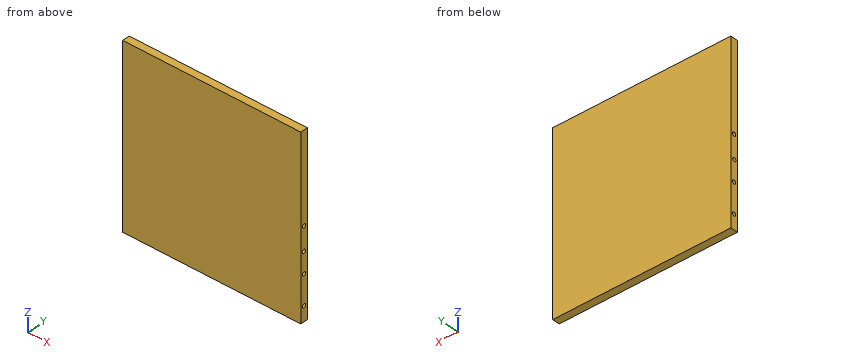
from build123d import *

# Parameters (mm, degrees)
SKETCH2_W               = 304.8
SKETCH2_H               = 304.8
BOSS_EXTRUDE1_DEPTH     = 12.7
SKETCH3_R               = 3.175
CUT_EXTRUDE1_DEPTH      = 343.16151121
SKETCH4_R               = 3.175
CUT_EXTRUDE2_DEPTH      = 343.16151121
CUT_EXTRUDE7_DEPTH      = 343.16151121
CUT_EXTRUDE7_DEPTH_BACK = 343.16151121
SKETCH5_R               = 3.175
CUT_EXTRUDE8_DEPTH      = 343.16151121
CUT_EXTRUDE8_DEPTH_BACK = 343.16151121
SKETCH6_R               = 3.175
SCALE1_SCALE            = 1.5


with BuildPart() as part:
    # Sketch2 → Boss-Extrude1 (new body)
    with BuildSketch(Plane(origin=(0, 0, 0), x_dir=(1, 0, 0), z_dir=(0, 1, 0))):
        with Locations((-98.332011444, 2.55215311)):
            Rectangle(SKETCH2_W, SKETCH2_H)
    extrude(amount=BOSS_EXTRUDE1_DEPTH)

    # Sketch3 → Cut-Extrude1 (cut, through all)
    with BuildSketch(Plane(origin=(54.067988556, 0, 0), x_dir=(0, 0, -1), z_dir=(1, 0, 0))):
        with Locations((2.55215311, 6.35)):
            Circle(SKETCH3_R)
    extrude(amount=-CUT_EXTRUDE1_DEPTH, mode=Mode.SUBTRACT)

    # Sketch4 → Cut-Extrude2 (cut, through all)
    with BuildSketch(Plane.ZY.offset(250.732011444)):
        with Locations((-42.726167629, 5.894382634)):
            Circle(SKETCH4_R)
    extrude(amount=-CUT_EXTRUDE2_DEPTH, mode=Mode.SUBTRACT)

    # Sketch5 → Cut-Extrude7 (cut, two sides: drawn at the far end of the back side and taken through both)
    with BuildSketch(Plane.ZY.offset(250.732011444).offset(-CUT_EXTRUDE7_DEPTH_BACK)):
        with Locations((-78.75215311, 6.35)):
            Circle(SKETCH5_R)
    extrude(amount=CUT_EXTRUDE7_DEPTH + CUT_EXTRUDE7_DEPTH_BACK, mode=Mode.SUBTRACT)

    # Sketch6 → Cut-Extrude8 (cut, two sides: drawn at the far end of the back side and taken through both)
    with BuildSketch(Plane.ZY.offset(250.732011444).offset(-CUT_EXTRUDE8_DEPTH_BACK)):
        with Locations((-129.55215311, 6.35)):
            Circle(SKETCH6_R)
    extrude(amount=CUT_EXTRUDE8_DEPTH + CUT_EXTRUDE8_DEPTH_BACK, mode=Mode.SUBTRACT)


with BuildPart() as part_1:
    # Scale1: scaled about (-98.332011444, 6.35385362, -0.493691098)
    add(part.part.scale(SCALE1_SCALE).moved(Location((49.166005722, -3.17692681, 0.246845549))))


solid = part_1.part
CAD build for the part. Positions are in the model's coordinates, mm. Round coordinates to 2 decimals unless told otherwise and drop trailing zeros. Write each loop counter-clockwise with the first axis right and the second up, starting at its lowest first coordinate (ties: lowest second). Pieces come first, ordered by that corner, then holes. Notation, with made-up numbers: M 24,46.25 L 81,46.25 A26 ccw 81,78.25 Z; hole C 7,48.25 d8. An arc over 180 degrees is marked long. Put each result on its own line as item: value. Start each with the question number.
1) Saw through at A-A, the plane x = 40. Write the cut outline in (y, z) (1 decimal), and give its area (3 significant figures).
2) Drill centre lines: probe 1 along Z at (x, y) = (29, 6.5); probe 2 along Z at (x, y) = (50.5, 5.5) (3 decimals). Where is each one in solid material? Low to high. Write a range as [from, to].
3) Pin check, flat tip, straight feed: pin 1 Ø7.5 at (y, z) = (5.66, -63.84) entering from -X. Stop position of the tip, or through.
Resolved:
1. outline: M -3.2,-232.2 L 15.9,-232.2 L 15.9,225 L -3.2,225 Z; hole C 5.7,-63.8 d9.5; hole C 6.3,-194.1 d9.5; hole C 6.3,-117.9 d9.5; hole C 6.3,-3.6 d9.5
1. area: 8,420 mm²
2. probe 1: [-232.18, -198.84], [-189.32, -122.64], [-113.12, -68.53], [-59.15, -8.34], [1.18, 225.02]
2. probe 2: [-232.181, -198.768], [-189.395, -122.568], [-113.195, -68.602], [-59.083, -8.268], [1.105, 225.019]
3. pin 1: through
